Read the model definition and answer for the solid it produces. Units are mm, in the model's axes. Coordinates: 2 decimals unless noted, no trailing zeros. Write each loop counter-clockwise with the first axis right and the second up, starting at its lowest first coordinate (ties: lowest second). Pieces come first, ordered by that corner, then holes. Notation, with made-up numbers: (-19.5, 34) -> (16.5, 34) arc R23 ccw to (16.5, 70) -> close; hole circle Ø6 at (-13.5, 33.5). An arc over 180 degrees is marked (long way). Answer in a Markdown table with one row per item. Add a question column.
Item 1: Section B-B on x = -5 is taken. Write down the section's boundary in (y, z), then the cut area to 3 significant figures.
Item 2: Section A-A on y = -23 is taken. Write down the section's boundary in (x, z), then the cut area to 3 significant figures.
Item 3: For a pull along X with two mould halves and no side action, classify faces 1 (the face through (-44.827, -0.369, 0.246)), 2 (the face through (43.3, 0.2, 0)) as +X half, -X half, draft (parallel to the pull), parting line (faces both ways), or undercut.
Item 4: Straight lines are drawn through the part: line 1 (Y direction, x = 0, z = 0.25); line 2 (Y direction, x = -23, z = 0.2); line 3 (X direction, y = -25, z = 0.25). For each, find the intervals that lie inside material, in ascending order. Write a range as from..to.
Item 5: Section C-C on y = 11.5 is taken. Write down the section's boundary in (x, z), then the cut area to 3 significant figures.
Autodesk Inventor part; units mm, degrees
ref_plane "YZ Plane" through (0, 0, 0) normal (1, 0, 0) x (0, 1, 0)
ref_plane "XZ Plane" through (0, 0, 0) normal (0, 1, 0) x (-1, 0, 0)
ref_plane "XY Plane" through (0, 0, 0) normal (0, 0, 1) x (1, 0, 0)
sketch "Sketch1" plane through (0, 0, 0) normal (0, 0, 1) x (1, 0, 0)
  circle A0 centre (39.8372, -23) radius 1.2295
  circle A1 centre (23, -39.8372) radius 1.2295
  circle A2 centre (0, -46) radius 1.2295
  circle A3 centre (-23, -39.8372) radius 1.2295
  circle A4 centre (-39.8372, -23) radius 1.2295
  circle A5 centre (-46, 0) radius 1.2295
  circle A6 centre (-39.8372, 23) radius 1.2295
  circle A7 centre (-23, 39.8372) radius 1.2295
  circle A8 centre (0, 46) radius 1.2295
  circle A9 centre (23, 39.8372) radius 1.2295
  circle A10 centre (39.8372, 23) radius 1.2295
  circle A11 centre (46, 0) radius 1.2295
  arc A12 (29.9143, -37.5385) -> (37.5385, -29.9143) centre (0, 0) ccw
  arc A13 (24.8949, -37.5114) -> (29.9143, -37.5385) centre (27.4214, -34.4103) ccw
  arc A14 (24.8949, -37.5114) -> (20.0383, -40.3153) centre (23, -39.8372) ccw
  arc A15 (17.5521, -44.6757) -> (20.0383, -40.3153) centre (16.0895, -40.9528) ccw
  arc A16 (7.1373, -47.4664) -> (17.5521, -44.6757) centre (0, 0) ccw
  arc A17 (2.8039, -44.9332) -> (7.1373, -47.4664) centre (6.5425, -43.5109) ccw
  arc A18 (2.8039, -44.9332) -> (-2.8039, -44.9332) centre (0, -46) ccw
  arc A19 (-7.1373, -47.4664) -> (-2.8039, -44.9332) centre (-6.5425, -43.5109) ccw
  arc A20 (-17.5521, -44.6757) -> (-7.1373, -47.4664) centre (0, 0) ccw
  arc A21 (-20.0383, -40.3153) -> (-17.5521, -44.6757) centre (-16.0895, -40.9528) ccw
  arc A22 (-20.0383, -40.3153) -> (-24.8949, -37.5114) centre (-23, -39.8372) ccw
  arc A23 (-29.9143, -37.5385) -> (-24.8949, -37.5114) centre (-27.4214, -34.4103) ccw
  arc A24 (-37.5385, -29.9143) -> (-29.9143, -37.5385) centre (0, 0) ccw
  arc A25 (-37.5114, -24.8949) -> (-37.5385, -29.9143) centre (-34.4103, -27.4214) ccw
  arc A26 (-37.5114, -24.8949) -> (-40.3153, -20.0383) centre (-39.8372, -23) ccw
  arc A27 (-44.6757, -17.5521) -> (-40.3153, -20.0383) centre (-40.9528, -16.0895) ccw
  arc A28 (-47.4664, -7.1373) -> (-44.6757, -17.5521) centre (0, 0) ccw
  arc A29 (-44.9332, -2.8039) -> (-47.4664, -7.1373) centre (-43.5109, -6.5425) ccw
  arc A30 (-44.9332, -2.8039) -> (-44.9332, 2.8039) centre (-46, 0) ccw
  arc A31 (-47.4664, 7.1373) -> (-44.9332, 2.8039) centre (-43.5109, 6.5425) ccw
  arc A32 (-44.6757, 17.5521) -> (-47.4664, 7.1373) centre (0, 0) ccw
  arc A33 (-40.3153, 20.0383) -> (-44.6757, 17.5521) centre (-40.9528, 16.0895) ccw
  arc A34 (-40.3153, 20.0383) -> (-37.5114, 24.8949) centre (-39.8372, 23) ccw
  arc A35 (-37.5385, 29.9143) -> (-37.5114, 24.8949) centre (-34.4103, 27.4214) ccw
  arc A36 (-29.9143, 37.5385) -> (-37.5385, 29.9143) centre (0, 0) ccw
  arc A37 (-24.8949, 37.5114) -> (-29.9143, 37.5385) centre (-27.4214, 34.4103) ccw
  arc A38 (-24.8949, 37.5114) -> (-20.0383, 40.3153) centre (-23, 39.8372) ccw
  arc A39 (-17.5521, 44.6757) -> (-20.0383, 40.3153) centre (-16.0895, 40.9528) ccw
  arc A40 (-7.1373, 47.4664) -> (-17.5521, 44.6757) centre (0, 0) ccw
  arc A41 (-2.8039, 44.9332) -> (-7.1373, 47.4664) centre (-6.5425, 43.5109) ccw
  arc A42 (-2.8039, 44.9332) -> (2.8039, 44.9332) centre (0, 46) ccw
  arc A43 (7.1373, 47.4664) -> (2.8039, 44.9332) centre (6.5425, 43.5109) ccw
  arc A44 (17.5521, 44.6757) -> (7.1373, 47.4664) centre (0, 0) ccw
  arc A45 (20.0383, 40.3153) -> (17.5521, 44.6757) centre (16.0895, 40.9528) ccw
  arc A46 (20.0383, 40.3153) -> (24.8949, 37.5114) centre (23, 39.8372) ccw
  arc A47 (29.9143, 37.5385) -> (24.8949, 37.5114) centre (27.4214, 34.4103) ccw
  arc A48 (37.5385, 29.9143) -> (29.9143, 37.5385) centre (0, 0) ccw
  arc A49 (37.5114, 24.8949) -> (37.5385, 29.9143) centre (34.4103, 27.4214) ccw
  arc A50 (37.5114, 24.8949) -> (40.3153, 20.0383) centre (39.8372, 23) ccw
  arc A51 (44.6757, 17.5521) -> (40.3153, 20.0383) centre (40.9528, 16.0895) ccw
  arc A52 (47.4664, 7.1373) -> (44.6757, 17.5521) centre (0, 0) ccw
  arc A53 (44.9332, 2.8039) -> (47.4664, 7.1373) centre (43.5109, 6.5425) ccw
  arc A54 (44.9332, 2.8039) -> (44.9332, -2.8039) centre (46, 0) ccw
  arc A55 (47.4664, -7.1373) -> (44.9332, -2.8039) centre (43.5109, -6.5425) ccw
  arc A56 (44.6757, -17.5521) -> (47.4664, -7.1373) centre (0, 0) ccw
  arc A57 (40.3153, -20.0383) -> (44.6757, -17.5521) centre (40.9528, -16.0895) ccw
  arc A58 (40.3153, -20.0383) -> (37.5114, -24.8949) centre (39.8372, -23) ccw
  arc A59 (37.5385, -29.9143) -> (37.5114, -24.8949) centre (34.4103, -27.4214) ccw
  circle A60 centre (0, 0) radius 49
extrude "Extrusion1" add sketch "Sketch1" along normal blind 0.5
properties part number "capsule.gasket"
Results below:
| question | item | result |
|---|---|---|
| 1 | outline | (-48.74, 0) -> (-47.2, 0) -> (-47.2, 0.5) -> (-48.74, 0.5) -> close; (47.2, 0) -> (48.74, 0) -> (48.74, 0.5) -> (47.2, 0.5) -> close |
| 1 | area | 1.54 mm2 |
| 2 | outline | (-43.27, 0) -> (-41.07, 0) -> (-41.07, 0.5) -> (-43.27, 0.5) -> close; (-38.61, 0) -> (-36.84, 0) -> (-36.84, 0.5) -> (-38.61, 0.5) -> close; (36.84, 0) -> (38.61, 0) -> (38.61, 0.5) -> (36.84, 0.5) -> close; (41.07, 0) -> (43.27, 0) -> (43.27, 0.5) -> (41.07, 0.5) -> close |
| 2 | area | 3.97 mm2 |
| 3 | face 1 | undercut |
| 3 | face 2 | draft |
| 4 | line 1 | y = -49..-47.23, -44.77..-43, 43..44.77, 47.23..49 |
| 4 | line 2 | y = -43.27..-41.07, -38.61..-36.84, 36.84..38.61, 41.07..43.27 |
| 4 | line 3 | x = -42.14..-37.59, 37.59..42.14 |
| 5 | outline | (-47.63, 0) -> (-46.6, 0) -> (-46.6, 0.5) -> (-47.63, 0.5) -> close; (46.6, 0) -> (47.63, 0) -> (47.63, 0.5) -> (46.6, 0.5) -> close |
| 5 | area | 1.03 mm2 |
